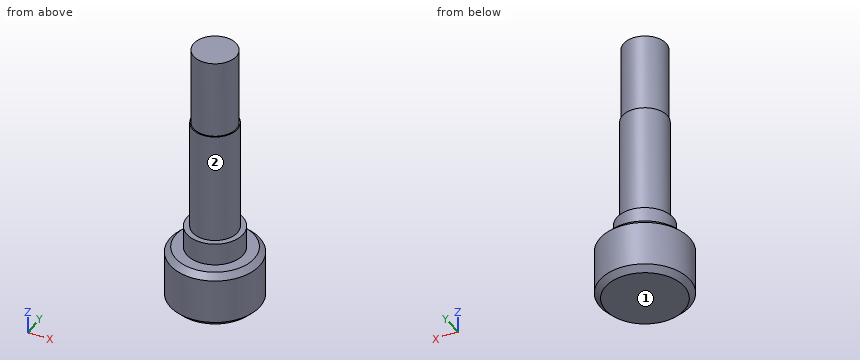
from build123d import *

# Parameters (mm, degrees)
SKETCH_1_R          = 4
EXTRUDE_1_DEPTH     = 5
SKETCH_2_R          = 2.5
EXTRUDE_2_DEPTH     = 2
SKETCH_3_R          = 2
EXTRUDE_3_DEPTH     = 17
CHAMFER_1_SIZE      = 0.5
CHAMFER_2_SIZE      = 0.5
CUT_EXTRUDE_START   = -7
SKETCH_4_R          = 2
SKETCH_4_R_2        = 1.9
CUT_EXTRUDE_1_DEPTH = 7


with BuildPart() as part:
    # 草图1 → 凸台-拉伸1 (new body)
    with BuildSketch(Plane.XY):
        Circle(SKETCH_1_R)
    extrude(amount=EXTRUDE_1_DEPTH)

    # 草图2 → 凸台-拉伸2 (add)
    with BuildSketch(Plane.XY.offset(5)):
        Circle(SKETCH_2_R)
    extrude(amount=EXTRUDE_2_DEPTH)

    # 草图3 → 凸台-拉伸3 (add)
    with BuildSketch(Plane.XY.offset(7)):
        Circle(SKETCH_3_R)
    extrude(amount=EXTRUDE_3_DEPTH)

    # 倒角1
    chamfer_1_edges = [part.edges().sort_by_distance(p)[0] for p in [
        (-4, 0, 0),
    ]]
    chamfer(chamfer_1_edges, length=CHAMFER_1_SIZE)

    # 倒角2
    chamfer_2_edges = [part.edges().sort_by_distance(p)[0] for p in [
        (-4, 0, 5),
    ]]
    chamfer(chamfer_2_edges, length=CHAMFER_2_SIZE)

    # 草图4 → 切除-拉伸1 (cut)
    with BuildSketch(Plane.XY.offset(24).offset(CUT_EXTRUDE_START)):
        Circle(SKETCH_4_R)
        Circle(SKETCH_4_R_2, mode=Mode.SUBTRACT)
    extrude(amount=CUT_EXTRUDE_1_DEPTH, mode=Mode.SUBTRACT)


solid = part.part
Can you work these out from the model? Positions are in its coordinate system, mm. Face numbers are marked on the shaded views. A direction names the side the tool comes from. Give positions to 0.01 mm unless a question says otherwise; leave off trailing zeros. Order: outer loops, then holes, each group sorted by start corner. A loop starts at its lowest first (then second) coordinate and runs counter-clockwise, first axis right, second up. Notation, with made-up numbers: M -29,-37.5 L -5,-37.5 A14 cw -5,-15.5 Z; hole C 53.5,18.5 d9. An arc over 180 degrees is marked long. Use one line per item in the form item = value.
Item 1: If I drill on line 1 along Z through (x, y) = (-3.25, 0.5); line 2 along Z through (x, y) = (0.5, 2.25); line 3 along X through (y, z) = (1.5, 6.75), over which ranges is the centre line in solid material (lowest first)? Write a range as [from, to].
Values follow:
line_1 = [0, 5]
line_2 = [0, 7]
line_3 = [-2, 2]
Item 2: For the marked faces 1 and 2, which set-ups out of +Z, -Z, +X, -X, +Y, -Y let a thin tool reach every point of the face, with its end or its side?
Values follow:
face_1 = -Z, +X, -X, +Y, -Y
face_2 = +Z
Item 3: If we section it at A-A, the plane y = 0: Write out the boundary of the cut face in (x, z).
Values follow:
outline = M -4,0.5 L -3.5,0 L 3.5,0 L 4,0.5 L 4,4.5 L 3.5,5 L 2.5,5 L 2.5,7 L 2,7 L 2,17 L 1.9,17 L 1.9,24 L -1.9,24 L -1.9,17 L -2,17 L -2,7 L -2.5,7 L -2.5,5 L -3.5,5 L -4,4.5 Z
Item 4: If we section it at D-D, the plane z = 3.25: Write out the boundary of the cut face in (x, y), and give its area (3 significant figures).
Values follow:
outline = C 0,0 d8
area = 50.3 mm^2
Item 5: If we section it at C-C, the plane z = 16.75: Write out the boundary of the cut face in (x, y), and give its area (3 significant figures).
Values follow:
outline = C 0,0 d4
area = 12.6 mm^2
Item 6: Will these pins go through, and if not, where does the flat tip stop? pin 1 Ø1.5 at (x, z) = (-1.5, 14) entering from -Y; pin 2 Ø4 at (x, z) = (-2.5, 6.5) entering from -Y.
Values follow:
pin_1 = -1.85
pin_2 = -3.44
